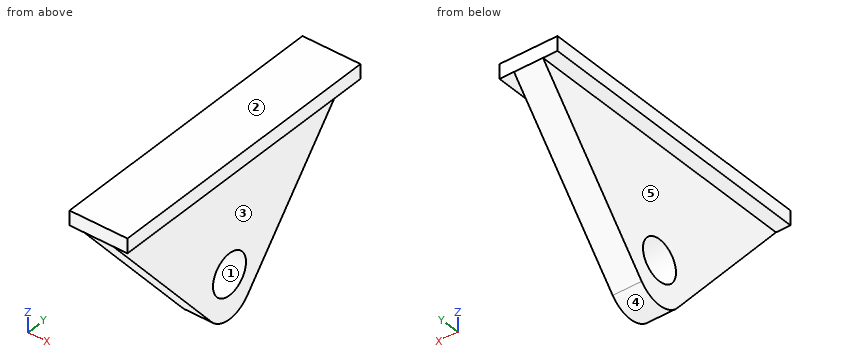
from build123d import *

# Parameters (mm, degrees)
SKETCH_1_W           = 12
SKETCH_1_H           = 60
EXTRUDE_1_DEPTH      = 3
EXTRUDE_2_DEPTH      = 3
EXTRUDE_2_DEPTH_BACK = 3
FILLET_1_R           = 6
SKETCH_4_R           = 4.25
CUT_EXTRUDE_1_DEPTH  = 46.029309177


with BuildPart() as part:
    # 草图1 → 凸台-拉伸1 (new body)
    with BuildSketch(Plane.XY):
        Rectangle(SKETCH_1_W, SKETCH_1_H)
    extrude(amount=EXTRUDE_1_DEPTH)

    # 草图3 → 凸台-拉伸2 (add, two sides: drawn at the far end of the back side and taken through both)
    with BuildSketch(Plane(origin=(0, 0, 0), x_dir=(0, 0, -1), z_dir=(1, 0, 0)).offset(-EXTRUDE_2_DEPTH_BACK)):
        Polygon((0, 30), (35.674118933, 0), (0, -30), align=None)
    extrude(amount=EXTRUDE_2_DEPTH + EXTRUDE_2_DEPTH_BACK)

    # 圆角1
    fillet_1_edges = [part.edges().sort_by_distance(p)[0] for p in [
        (0, 0, -35.674118933),
    ]]
    fillet(fillet_1_edges, radius=FILLET_1_R)

    # 草图4 → 切除-拉伸1 (cut, through all)
    with BuildSketch(Plane.ZY.offset(3)):
        with Locations((-23.257154685, 0)):
            Circle(SKETCH_4_R)
    extrude(amount=-CUT_EXTRUDE_1_DEPTH, mode=Mode.SUBTRACT)


solid = part.part
Build history of the part. All positions in model axes, mm. Face numbers are marked on the shaded views. A direction names the side the tool comes from. Give positions to 0.01 mm unless a question says otherwise; leave off trailing zeros. Order: outer loops, then holes, each group sorted by start corner. A loop starts at its lowest first (then second) coordinate and runs counter-clockwise, first axis right, second up. Notation, with made-up numbers: M 26.5,-13 L 30.5,-13 A9 ccw 30.5,-3 Z; hole C -3,-0.5 d7. An arc over 180 degrees is marked long. Use one line per item in the form item = value.
Q1. Slice it at B-B, the plane x = -2. Write the cut outline in (y, z).
Conclusion:
outline = M -30,0 L -4.59,-30.21 A6 ccw 4.59,-30.21 L 30,0 L 30,3 L -30,3 Z; hole C 0,-23.26 d8.5
Q2. Pull direction Z, two halves, no side cores. Call the marked faces 1, 2 and 3: released by +Z, released by -Z, zero draft, split by the parting line, or undercut.
Conclusion:
face_1 = undercut
face_2 = released by +Z
face_3 = zero draft
Q3. Pin check, flat tips, straight feed: P1, Ø1, axis at y = -9, z = -21, coming from the +X side; P2, Ø1, axis at x = 1.5, y = 20.5, coming from the -Z side; P3, Ø13.5, axis at y = 0, z = -23.26, coming from the -X side. Stop position of each tip, or through.
Conclusion:
P1 = 3
P2 = -11.89
P3 = -3
Q4. Which spindle directions (+Z, -Z, +X, -X, +Y, -Y) get a long thin tool onto all of the face, cutting with end or side? Do the marked faces 4 and 5. Say none if no direction does.
Conclusion:
face_4 = -Z, +X, -X
face_5 = -Z, -X, +Y, -Y
Q5. Slice it at C-C, the plane z = -25.5. Write the cut outline in (x, y).
Conclusion:
outline = M -3,-8.56 L 3,-8.56 L 3,-3.61 L -3,-3.61 Z; M -3,3.61 L 3,3.61 L 3,8.56 L -3,8.56 Z
Q6. Slice it at A-A, the plane y = 0. Write the cut outline in (x, z).
Conclusion:
outline = M -6,0 L -3,0 L -3,-19.01 L 3,-19.01 L 3,0 L 6,0 L 6,3 L -6,3 Z; M -3,-32.35 L 3,-32.35 L 3,-27.51 L -3,-27.51 Z
Q7. Wall check: probe 1 along X at (y, z) = (-3, -8); probe 2 along Y at (x, z) = (1.5, -26.5); probe 3 along Z at (x, y) = (-4.25, -20). Give the ranges that are in metal, low to high.
Conclusion:
probe_1 = -3 to 3
probe_2 = -7.71 to -2.75, 2.75 to 7.71
probe_3 = 0 to 3
Q8. Slice it at D-D, the plane y = -6.5. Write the cut outline in (x, z), and give its area (3 significant figures).
Conclusion:
outline = M -6,0 L -3,0 L -3,-27.94 L 3,-27.94 L 3,0 L 6,0 L 6,3 L -6,3 Z
area = 204 mm2
